Could you check a few things on this model? Use its own coordinates, in mm. Round coordinates to 2 decimals unless told otherwise and drop trailing zeros. Loops run counter-clockwise (first coordinate to the right, second up) from the corner with the lowest first, then second, coordinate; pieces in that order, holes last. Notation, with made-up numbers: M 75,41 L 104,41 A29 ccw 104,64 Z; hole C 19.5,87 d7. An arc over 180 degrees is marked long. Return JSON: item names as keys, results as strings. Group by question number.
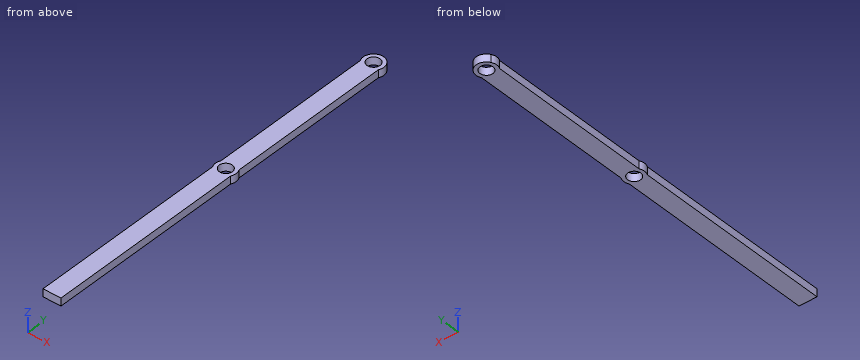
```python
from build123d import *

# Parameters (mm, degrees)
SKETCH2_R           = 20
SKETCH2_R_2         = 12.7
BOSS_EXTRUDE1_DEPTH = 7.5
SKETCH4_W           = 35
SKETCH4_H           = 15
BOSS_EXTRUDE2_DEPTH = 400
SKETCH4_2_W         = 35
SKETCH4_2_H         = 15
BOSS_EXTRUDE3_DEPTH = 350
SKETCH5_R           = 12.7
CUT_EXTRUDE1_DEPTH  = 8.5
LPATTERN1_COUNT     = 2
LPATTERN1_PITCH     = 340


with BuildPart() as part:
    # Sketch2 → Boss-Extrude1 (new body, symmetric)
    with BuildSketch(Plane.XY):
        Circle(SKETCH2_R)
        Circle(SKETCH2_R_2, mode=Mode.SUBTRACT)
    boss_extrude1 = extrude(amount=BOSS_EXTRUDE1_DEPTH, both=True)

    # Sketch4 → Boss-Extrude2 (add)
    with BuildSketch(Plane(origin=(0, 0, 0), x_dir=(1, 0, 0), z_dir=(0, 1, 0))):
        Rectangle(SKETCH4_W, SKETCH4_H)
    extrude(amount=-BOSS_EXTRUDE2_DEPTH)

    # Sketch4<2> → Boss-Extrude3 (add)
    with BuildSketch(Plane(origin=(0, 0, 0), x_dir=(1, 0, 0), z_dir=(0, 1, 0))):
        Rectangle(SKETCH4_2_W, SKETCH4_2_H)
    extrude(amount=BOSS_EXTRUDE3_DEPTH)

    # Sketch5 → Cut-Extrude1 (cut, symmetric)
    with BuildSketch(Plane.XY):
        Circle(SKETCH5_R)
    cut_extrude1 = extrude(amount=CUT_EXTRUDE1_DEPTH, both=True, mode=Mode.SUBTRACT)

    # LPattern1: Boss-Extrude1, Cut-Extrude1 ×2
    with Locations(*[(0, i * LPATTERN1_PITCH, 0) for i in range(1, LPATTERN1_COUNT)]):
        add(boss_extrude1)
        add(cut_extrude1, mode=Mode.SUBTRACT)


solid = part.part
```
1. I'm going to push flat-ended pins straight in: pin 1 Ø8 at (x, z) = (-9.5, -1.5) entering from +Y; pin 2 Ø8 at (y, z) = (230, -5.5) entering from -X; pin 3 Ø7.5 at (y, z) = (-118, -2) entering from +X. Where does each tip first touch, or does it pass through?
2. I need wall thicknesses on probe 1 along Y at (x, z) = (0, -1); probe 2 along Y at (x, z) = (-4, 3.5); probe 3 along X at (y, z) = (340, 2.75). Which ranges of each line are inside material? Lowest first, please.
3. If we section it at C-C, the plane z = 1.25: Please give me the cut outline in (x, y).
4. If we section it at A-A, the plane x = 0: Please give me the cut outline in (y, z), then the cut area to 3 significant figures.
5. If we section it at B-B, the plane y = 340: Please give me the cut outline in (x, z), then the cut area to 3 significant figures.
6. If we section it at D-D, the plane y = 90: Please give me the cut outline in (x, z).
Geometry results:
{
 "1": {"pin 1": "y = 359.23", "pin 2": "x = -17.5", "pin 3": "x = 17.5"},
 "2": {"probe 1": "-400 to -12.7, 12.7 to 327.3, 352.7 to 360", "probe 2": "-400 to -12.05, 12.05 to 327.95, 352.05 to 359.6", "probe 3": "-20 to -12.7, 12.7 to 20"},
 "3": {"outline": "M -17.5,-400 L 17.5,-400 L 17.5,-9.68 A20 ccw 17.5,9.68 L 17.5,330.32 A20 ccw 17.5,349.68 L 17.5,350 L 17.32,350 A20 ccw -17.32,350 L -17.5,350 L -17.5,349.68 A20 ccw -17.5,330.32 L -17.5,9.68 A20 ccw -17.5,-9.68 Z; hole C 0,0 d25.4; hole C 0,340 d25.4"},
 "4": {"outline": "M -400,-7.5 L -12.7,-7.5 L -12.7,7.5 L -400,7.5 Z; M 12.7,-7.5 L 327.3,-7.5 L 327.3,7.5 L 12.7,7.5 Z; M 352.7,-7.5 L 360,-7.5 L 360,7.5 L 352.7,7.5 Z", "area": "10,600 mm^2"},
 "5": {"outline": "M -20,-7.5 L -12.7,-7.5 L -12.7,7.5 L -20,7.5 Z; M 12.7,-7.5 L 20,-7.5 L 20,7.5 L 12.7,7.5 Z", "area": "219 mm^2"},
 "6": {"outline": "M -17.5,-7.5 L 17.5,-7.5 L 17.5,7.5 L -17.5,7.5 Z"}
}
